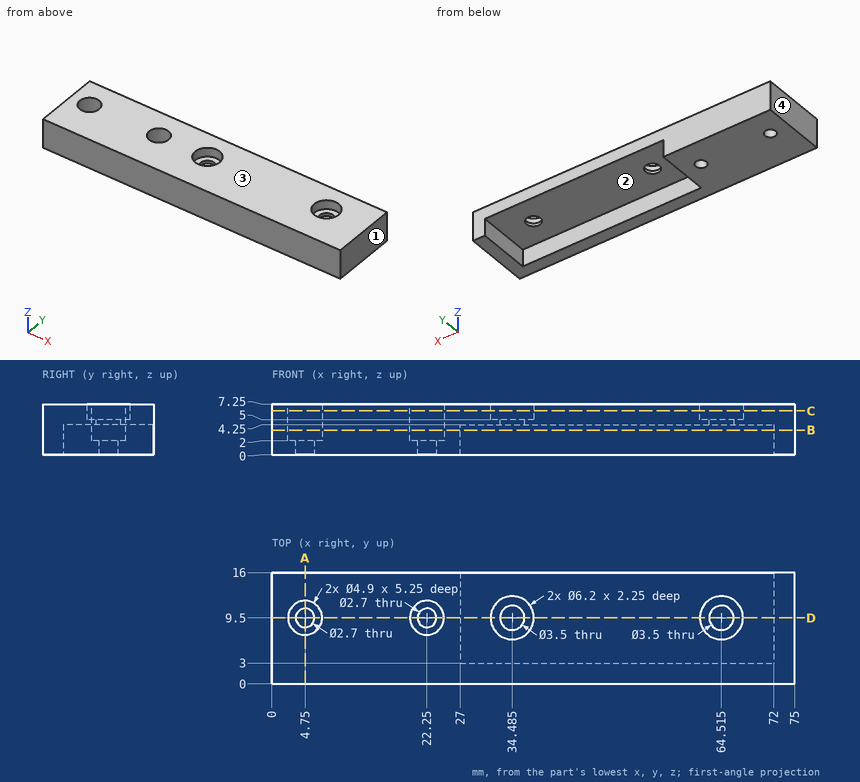
Check sheet for the drawn part. Datum: minimum x, y, z corner. Units: mm. Give positions to 0.01 mm unless a question says otherwise; leave off trailing zeros. Write each loop counter-clockwise with the first axis right and the second up, starting at its lowest first coordinate (ties: lowest second). Pieces come first, ordered by that corner, then holes.
(1) Cross-section at A-A (x = 4.75). Enter the section's corners in (y, z), plus the area to 3 significant figures.
(2) Cross-section at C-C (z = 6.25). Enter the section's corners in (x, y) (3 decimals), plus the area to 3 significant figures.
(3) Cross-section at D-D (y = 9.5). State how many separate pieces and enclosed holes the cut face has, plus the area to 3 significant figures.
(4) Cross-section at B-B (z = 3.5). Enter the section's corners in (x, y), plus the area to 3 significant figures.
(5) Gauge pin test, flat ends, axial feed: pin 1 (4 mm diameter, centred on x = 4.75, y = 9.5, fed in from +Z); pin 2 (8 mm diameter, centred on x = 34.485, y = 9.5, fed in from -Z); pin 3 (1.9 mm diameter, centred on x = 35, y = 10.5, fed in from +Z). Record the tip position at first contact, or that the pin passes through.
(6) Mould release check, pull along X, two halves, no side actions. Record for the marked faces 1, 2, 3 and 4: +X half, -X half, draft (parallel to the pull), parting line (faces both ways), or undercut.
(7) Material ranges on line 1 (Y direction, x = 22.25, z = 5.6); line 2 (X direction, y = 5, z = 2.25); line 3 (Z direction, x = 64, y = 4), recorded low to high.
Worked out:
1. outline: (0, 0) - (8.15, 0) - (8.15, 2) - (7.05, 2) - (7.05, 7.25) - (0, 7.25) - close; (10.85, 0) - (16, 0) - (16, 7.25) - (11.95, 7.25) - (11.95, 2) - (10.85, 2) - close
1. area: 84.9 mm2
2. outline: (0, 0) - (75, 0) - (75, 16) - (0, 16) - close; hole circle Ø4.9 at (4.75, 9.5); hole circle Ø4.9 at (22.25, 9.5); hole circle Ø6.2 at (34.485, 9.5); hole circle Ø6.2 at (64.515, 9.5)
2. area: 1,100 mm2
3. separate pieces: 5
3. enclosed holes: 0
3. area: 257 mm2
4. outline: (0, 0) - (75, 0) - (75, 16) - (72, 16) - (72, 3) - (27, 3) - (27, 16) - (0, 16) - close; hole circle Ø4.9 at (4.75, 9.5); hole circle Ø4.9 at (22.25, 9.5)
4. area: 577 mm2
5. pin 1: stops at z = 2
5. pin 2: stops at z = 4.25
5. pin 3: stops at z = 5
6. face 1: +X half
6. face 2: undercut
6. face 3: draft
6. face 4: -X half
7. line 1: y = 0 to 7.05, 11.95 to 16
7. line 2: x = 0 to 27, 72 to 75
7. line 3: z = 4.25 to 7.25
